from build123d import *

# Parameters (mm, degrees)
SKETCH_1_W      = 30
SKETCH_1_H      = 100
SKETCH_2_W      = 30
SKETCH_2_H      = 60
EXTRUDE_1_DEPTH = 100
FILLET_1_R      = 30


with BuildPart() as part:
    # Эскиз1 → Повернуть1 (revolve)
    with BuildSketch(Plane.XY, mode=Mode.PRIVATE) as revolve_1_sk:
        with Locations((-15, 50)):
            Rectangle(SKETCH_1_W, SKETCH_1_H)
    revolve(revolve_1_sk.sketch.rotate(Axis((0, 0, 0), (0, 1, 0)), 270), axis=Axis((0, 0, 0), (0, 1, 0)))

    # Эскиз2 → Бобышка-Вытянуть1 (add)
    with BuildSketch(Plane(origin=(0, 100, 0), x_dir=(1, 0, 0), z_dir=(0, 1, 0))):
        with Locations((-15, 0)):
            Rectangle(SKETCH_2_W, SKETCH_2_H)
    extrude(amount=EXTRUDE_1_DEPTH)

    # Скругление1
    fillet_1_edges = [part.edges().sort_by_distance(p)[0] for p in [
        (-30, 150, -30),
    ]]
    fillet(fillet_1_edges, radius=FILLET_1_R - 0.0001)  # a hair under: the kernel refuses the full size
    fillet_1_2_edges = [part.edges().sort_by_distance(p)[0] for p in [
        (-30, 150, 30),
    ]]
    fillet(fillet_1_2_edges, radius=FILLET_1_R - 0.0001)  # a hair under: the kernel refuses the full size
    fillet_1_3_edges = [part.edges().sort_by_distance(p)[0] for p in [
        (-30, 200, 0),
    ]]
    fillet(fillet_1_3_edges, radius=FILLET_1_R - 0.0001)  # a hair under: the kernel refuses the full size


solid = part.part
Read the model definition and answer for the solid it produces. Units are mm, in the model's axes. A direction names the side the tool comes from. Round coordinates to 2 decimals unless told otherwise and drop trailing zeros. Use a Markdown table: item, result.
(1) Which of the six approach directions +Z, -Z, +X, -X, +Y, -Y give full straight-line access (tool end or side, diameter ignored) to faces 1 (the flat face through (0, 149, 0)), 2 (the cylindrical face through (-1.32, 50.7, 29.97))?
Reported:
| item | result |
|---|---|
| face 1 | +Z, -Z, +X, +Y |
| face 2 | +Y, -Y |
(2) Each of these flat-tipped pins is pushed along its axis until it touches: pin 1 Ø10 at (y, z) = (70.5, -15) entering from +X; pin 2 Ø5 at (x, z) = (6, -18) entering from -Y; pin 3 Ø2 at (x, z) = (-21.5, 3) entering from +Y; pin 4 Ø2 at (y, z) = (105, 9.5) entering from +X. Where does it stop, or does it pass through?
Reported:
| item | result |
|---|---|
| pin 1 | x = 28.28 |
| pin 2 | y = 0 |
| pin 3 | y = 191.71 |
| pin 4 | x = 0 |
(3) Straight lines are drawn through the part: line 1 along Y through (x, z) = (21, -9.5); line 2 along Z through (x, y) = (1, 79.5); line 3 along X through (y, z) = (184, -7). For each, find the intervals that lie inside material, in ascending order. Write a range as [from, to].
Reported:
| item | result |
|---|---|
| line 1 | [0, 100] |
| line 2 | [-29.98, 29.98] |
| line 3 | [-25.59, 0] |
